from build123d import *

# Parameters (mm, degrees)
SKETCH1_R           = 4
BOSS_EXTRUDE1_DEPTH = 50
BOSS_EXTRUDE2_START = -23
SKETCH2_R           = 6
BOSS_EXTRUDE2_DEPTH = 5


with BuildPart() as part:
    # Sketch1 → Boss-Extrude1 (new body)
    with BuildSketch(Plane(origin=(0, 0, 0), x_dir=(1, 0, 0), z_dir=(0, 1, 0))):
        with Locations(Location((0, 0, 0), (0, 0, 270))):
            Circle(SKETCH1_R)
    extrude(amount=BOSS_EXTRUDE1_DEPTH)

    # Sketch2 → Boss-Extrude2 (add)
    with BuildSketch(Plane(origin=(0, 50, 0), x_dir=(1, 0, 0), z_dir=(0, 1, 0)).offset(BOSS_EXTRUDE2_START)):
        with Locations(Location((0, 0, 0), (0, 0, 270))):
            Circle(SKETCH2_R)
    extrude(amount=-BOSS_EXTRUDE2_DEPTH)


solid = part.part
Design review of the part built by this model. Coordinates are the model's own, in mm. A direction names the side the tool comes from. Round coordinates to 2 decimals unless told otherwise and drop trailing zeros. Write each loop counter-clockwise with the first axis right and the second up, starting at its lowest first coordinate (ties: lowest second). Pieces come first, ordered by that corner, then holes. Notation, with made-up numbers: M -26,-22.5 L 5,-22.5 A14 cw 5,1.5 Z; hole C 40.25,32.5 d5. An arc over 180 degrees is marked long. One line per item, written item: value. Start each with the question number.
1. Clearance check with flat-ended pins moving along their axes: P1, Ø6, axis at x = -4, y = 27, coming from the -Z side; P2, Ø3, axis at y = 29, z = 3.5, coming from the +X side; P3, Ø3, axis at y = 11.5, z = 0, coming from the +X side. State where each tip first meets the part, or that it passes through.
2. Take a section at D-D on y = 5. State the section outline as (x, z) points, then the cut area to 3 significant figures.
3. To check wall thickness, follow probe 1 along Y at (x, z) = (-4, 3.5); probe 2 along X at (y, z) = (6.5, 0.25); probe 3 along X at (y, z) = (9, -0.75). State the ranges of each line that lie inside material, in increasing order. Write a range as from..to.
4. For faces 1 (the face through (1.802, 24.535, 5.723)), 2 (the face through (-3.905, 10.846, -0.867)), 3 (the face through (-3.92, 27, -1.42)), list the 3-axis set-ups (+Z, -Z, +X, -X, +Y, -Y) from which the entire face can be reached by the end or side of a thin tool; tool diameter is ignored.
5. Take a section at B-B on z = 0. State the section outline as (x, y) points.
6. Take a section at A-A on x = 0. State the section outline as (y, z) points, then the cut area to 3 significant figures.
7. Take a section at C-C on y = 23. State the section outline as (x, z) points, then the cut area to 3 significant figures.
Computed:
1. P1: stops at z = -5.92
1. P2: stops at x = 3.46
1. P3: stops at x = 4
2. outline: C 0,0 d8
2. area: 50.3 mm²
3. probe 1: y = 22..27
3. probe 2: x = -3.99..3.99
3. probe 3: x = -3.93..3.93
4. face 1: +Y, -Y
4. face 2: -Y
4. face 3: +Y
5. outline: M -6,22 L -4,22 L -4,0 L 4,0 L 4,22 L 6,22 L 6,27 L 4,27 L 4,50 L -4,50 L -4,27 L -6,27 Z
6. outline: M 0,-4 L 22,-4 L 22,-6 L 27,-6 L 27,-4 L 50,-4 L 50,4 L 27,4 L 27,6 L 22,6 L 22,4 L 0,4 Z
6. area: 420 mm²
7. outline: C 0,0 d12
7. area: 113 mm²
